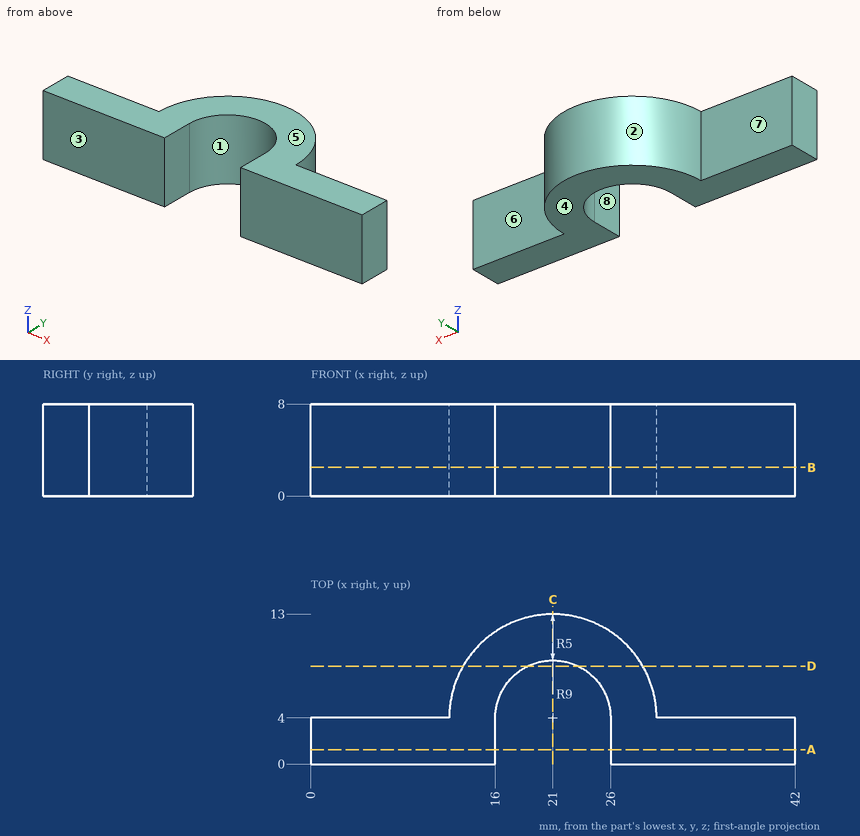
Can you work these out from the drawing? Everything is in mm from the part's minimum corner. A direction names the side the tool comes from. Coordinates: 2 decimals unless noted, no trailing zeros. Loops run counter-clockwise (first coordinate to the right, second up) from the corner with the lowest first, then second, coordinate; pieces in that order, holes last. Notation, with made-up numbers: (-20, 55.5) - (-10, 55.5) arc R23 cw to (-10, 88.5) - close; hole circle Ø10 at (28.5, 26.25). An arc over 180 degrees is marked (long way). Answer as CSV lines item,"result".
Q1. For the marked faces 4, 5, 6, 7 and 8, which set-ups out of +Z, -Z, +X, -X, +Y, -Y let a thin tool reach every point of the face, with its end or its side?
Response:
face 4,"-Z, +X, -X, +Y, -Y"
face 5,"+Z, +X, -X, +Y, -Y"
face 6,"+Z, -Z, +X, +Y"
face 7,"+Z, -Z, -X, +Y"
face 8,"+Z, -Z, -Y"
Q2. We'd pull the mould along X, two halves only. Please class the marked faces 1, 2 and 3: pulls with the +X half, pulls with the -X half, needs draft (parallel to the pull), parting line crosses it, or undercut.
Response:
face 1,"undercut"
face 2,"parting line crosses it"
face 3,"needs draft"
Q3. If we section it at D-D, the plane y = 8.5: Write out the boundary of the cut face in (x, z), and give its area (3 significant figures).
Response:
outline,"(13.21, 0) - (18.82, 0) - (18.82, 8) - (13.21, 8) - close; (23.18, 0) - (28.79, 0) - (28.79, 8) - (23.18, 8) - close"
area,"89.8 mm2"
Q4. If we section it at B-B, the plane z = 2.5: Write out the boundary of the cut face in (x, y).
Response:
outline,"(0, 0) - (16, 0) - (16, 4) arc R5 cw to (26, 4) - (26, 0) - (42, 0) - (42, 4) - (30, 4) arc R9 ccw to (12, 4) - (0, 4) - close"
Q5. If we section it at A-A, the plane y = 1.25: Write out the boundary of the cut face in (x, z), and give its area (3 significant figures).
Response:
outline,"(0, 0) - (16, 0) - (16, 8) - (0, 8) - close; (26, 0) - (42, 0) - (42, 8) - (26, 8) - close"
area,"256 mm2"
Q6. If we section it at C-C, the plane x = 21: Write out the boundary of the cut face in (y, z).
Response:
outline,"(9, 0) - (13, 0) - (13, 8) - (9, 8) - close"
Q7. If I drill on L1, parallel to X at y = 1.5, z = 4.25; L2, parallel to Y at x = 10.5, z = 4.75; L3, parallel to X at y = 4.5, z = 7, over which ranges is the centre line in solid material (lowest first)? Write a range as [from, to].
Response:
L1,"[0, 16], [26, 42]"
L2,"[0, 4]"
L3,"[12.01, 16.03], [25.97, 29.99]"
Q8. For pin 1 (1.5 mm diameter, centred on y = 8, z = 7, fed in from -X); pin 2 (3 mm diameter, centred on y = 11.5, z = 7, fed in from +X); pin 3 (4 mm diameter, centred on y = 6.5, z = 4, fed in from +X), each with a flat end and sliding along its axis, tell me the tip position at first contact or that it passes through.
Response:
pin 1,"x = 12.61"
pin 2,"x = 27.71"
pin 3,"x = 29.99"
